Geometry: final body of the model. Coordinates: model frame, mm. A direction names the side the tool comes from. Round coordinates to 2 decimals unless told otherwise and drop trailing zeros. Write each loop counter-clockwise with the first axis right and the second up, starting at its lowest first coordinate (ties: lowest second). Pieces come first, ordered by that corner, then holes. Notation, with made-up numbers: M 15.5,51.25 L 31.5,51.25 A23 ccw 31.5,81.25 Z; hole C -0.5,74.25 d5. An arc over 180 degrees is marked long. Use one line per item in the form item = value. Start each with the question number.
Item 1: Pull-direction query (Y, two-part tool) for faces 3 (the flat face through (33.401, 114, 2)), 4 (the flat face through (0, 63, 2)), 5 (the flat face through (63, 0, 2)), 6 (the flat face through (63, 127, 2)); classes: pulls with the +Y half, pulls with the -Y half, needs draft (parallel to the pull), parting line crosses it, or undercut.
Item 2: Ray query, probe 1 along X at (y, z) = (47.5, 2.5); probe 2 along Y at (x, z) = (68, 0.25); probe 3 along X at (y, z) = (21, 1.95). Return the intervals inside material, ascending.
Item 3: Section query A-A (y = 28.5). Return loops of the section in (x, z) (3 decimals), and give its area (3 significant figures).
Item 4: Reachability of faces 1 (the flat face through (63, 63, 3.175)), 2 (the flat face through (64, 114.3, 2)) from +Z, -Z, +X, -X, +Y, -Y: full face, straight path, thin tool, end or side. Return the list, or none.
from build123d import *

# Parameters (mm, degrees)
F0_W     = 127
F0_H     = 3.175
F1_DEPTH = 127
F3_DEPTH = 25
F4_R     = 1.5


with BuildPart() as f1:
    # F0 (on Front) → F1 (new body)
    with BuildSketch(Plane.XZ):
        with Locations((63.5, 1.5875)):
            Rectangle(F0_W, F0_H)
    extrude(amount=-F1_DEPTH)

    # F2 (on face) → F3 (cut)
    with BuildSketch(Plane.XY.offset(3.175)):
        Polygon((33.401, 106.299), (33.401, 122.301), (17.399, 122.301), (17.399, 106.299), (22.4, 106.299), (22.4, 12.7), (28.4, 12.7), (47.8, 12.7), (53.8, 12.7), (53.8, 104.3), (73.2, 104.3), (73.2, 12.7), (79.2, 12.7), (98.6, 12.7), (104.6, 12.7), (104.6, 106.299), (109.601, 106.299), (109.601, 122.301), (93.599, 122.301), (93.599, 106.299), (98.6, 106.299), (98.6, 22.7), (79.2, 22.7), (79.2, 114.3), (73.2, 114.3), (53.8, 114.3), (47.8, 114.3), (47.8, 22.7), (28.4, 22.7), (28.4, 106.299), align=None)
    extrude(amount=-F3_DEPTH, mode=Mode.SUBTRACT)

    # F4
    f4_edges = [f1.edges().sort_by_distance(p)[0] for p in [
        (17.399, 122.301, 1.5875),
        (33.401, 122.301, 1.5875),
        (17.399, 106.299, 1.5875),
        (22.4, 106.299, 1.5875),
        (28.4, 106.299, 1.5875),
        (33.401, 106.299, 1.5875),
        (53.8, 104.3, 1.5875),
        (73.2, 104.3, 1.5875),
        (98.6, 106.299, 1.5875),
        (104.6, 106.299, 1.5875),
        (104.6, 12.7, 1.5875),
        (79.2, 22.7, 1.5875),
        (28.4, 22.7, 1.5875),
        (53.8, 12.7, 1.5875),
        (47.8, 22.7, 1.5875),
        (98.6, 22.7, 1.5875),
        (73.2, 12.7, 1.5875),
        (22.4, 12.7, 1.5875),
        (109.601, 122.301, 1.5875),
        (79.2, 114.3, 1.5875),
        (47.8, 114.3, 1.5875),
        (93.599, 122.301, 1.5875),
        (109.601, 106.299, 1.5875),
        (93.599, 106.299, 1.5875),
    ]]
    fillet(f4_edges, radius=F4_R)


solid = f1.part
Working result:
q1.face_3 = undercut
q1.face_4 = needs draft
q1.face_5 = pulls with the -Y half
q1.face_6 = pulls with the +Y half
q2.probe_1 = 0 to 22.4, 28.4 to 47.8, 53.8 to 73.2, 79.2 to 98.6, 104.6 to 127
q2.probe_2 = 0 to 104.3, 114.3 to 127
q2.probe_3 = 0 to 22.4, 53.8 to 73.2, 104.6 to 127
q3.outline = M 0,0 L 22.4,0 L 22.4,3.175 L 0,3.175 Z; M 28.4,0 L 47.8,0 L 47.8,3.175 L 28.4,3.175 Z; M 53.8,0 L 73.2,0 L 73.2,3.175 L 53.8,3.175 Z; M 79.2,0 L 98.6,0 L 98.6,3.175 L 79.2,3.175 Z; M 104.6,0 L 127,0 L 127,3.175 L 104.6,3.175 Z
q3.area = 327 mm²
q4.face_1 = +Z, +X, -X, +Y, -Y
q4.face_2 = +Z, -Z
